Work out the finished part from the listing and answer in its coordinate system (mm). Give positions to 0.01 mm unless a question says otherwise; leave off trailing zeros. Loops run counter-clockwise (first coordinate to the right, second up) from the corner with the lowest first, then second, coordinate; pieces in that order, holes last.
from build123d import *

# Parameters (mm, degrees)
PAD013_DEPTH         = 9.4
POCKET039_DEPTH      = 100
POCKET039_DEPTH_BACK = 100
SKETCH049_R          = 2.3
POCKET040_DEPTH      = 1.101
CHAMFER010_SIZE      = 0.5


with BuildPart() as part:
    # Sketch047 (on Face1 of ShapeBinder008) → Pad013 (new body)
    with BuildSketch(Plane.XY.offset(4.85)):
        Polygon((-4.5, -10), (-5.6, -11.1), (5.6, -11.1), (4.5, -10), align=None)
    extrude(amount=-PAD013_DEPTH)

    # Sketch048 (on DatumPlane) → Pocket039 (cut, two sides)
    with BuildSketch(Plane(origin=(-4.866667, -10.366667, 1.716667), x_dir=(0, -1, 0), z_dir=(-1, 0, 0))) as pocket039_sk:
        Polygon((0.833333, 2.591912), (-0.366667, 1.391912), (-1.166667, 1.391912), (-1.166667, 3.391912), (0.833333, 3.391912), align=None)
    extrude(amount=-POCKET039_DEPTH, mode=Mode.SUBTRACT)
    extrude(pocket039_sk.sketch, amount=POCKET039_DEPTH_BACK, mode=Mode.SUBTRACT)

    # Sketch049 (on Face5 of Pocket039) → Pocket040 (cut, through all)
    with BuildSketch(Plane(origin=(0, -10, 0), x_dir=(-1, 0, 0), z_dir=(0, 1, 0))):
        with Locations((0, 1.15)):
            Circle(SKETCH049_R)
    extrude(amount=-POCKET040_DEPTH, mode=Mode.SUBTRACT)

    # Chamfer010
    chamfer010_edges = [part.edges().sort_by_distance(p)[0] for p in [
        (0, -10, -4.55),
    ]]
    chamfer(chamfer010_edges, length=CHAMFER010_SIZE)


solid = part.part
Item 1: Find section B-B, the plane x = 0.75. Write down the section's boundary in (y, z), plus the area to 3 significant figures.
Item 2: Determine the mould class of faces 1 (the face through (0.499, -10.542, -1.095)), 2 (the face through (1.1, -10, -1.2)), 3 (the face through (5.1, -10.6, -0.1)) for opening direction X: released by +X, released by -X, zero draft, split by the parting line, or undercut.
Item 3: Find section C-C, the plane y = -10.95. Write down the section's boundary in (x, z), plus the area to 3 significant figures.
Item 4: Consider line 1 (X direction, y = -10.5, z = 1.15); line 2 (Z direction, x = 0, y = -10.75); line 3 (X direction, y = -10.85, z = 1.15). Determine where each line is inside the solid, lowest interval first.
Item 5: Find section D-D, the plane x = -4. Write down the section's boundary in (y, z).
Item 6: Find section A-A, the plane z = 1.15. Write down the section's boundary in (x, y), plus the area to 3 significant figures.
Ans:
1. outline: (-11.1, -4.55) - (-10.5, -4.55) - (-10, -4.05) - (-10, -1.02) - (-11.1, -1.02) - close; (-11.1, 3.32) - (-10.22, 3.32) - (-11.1, 4.21) - close
1. area: 4.14 mm2
2. face 1: undercut
2. face 2: zero draft
2. face 3: released by +X
3. outline: (-5.45, -4.55) - (5.45, -4.55) - (5.45, 4.06) - (-5.45, 4.06) - close; hole circle Ø4.6 at (0, 1.15)
3. area: 77.2 mm2
4. line 1: x = -5 to -2.3, 2.3 to 5
4. line 2: z = -4.55 to -1.15, 3.45 to 3.86
4. line 3: x = -5.35 to -2.3, 2.3 to 5.35
5. outline: (-11.1, -4.55) - (-10.5, -4.55) - (-10, -4.05) - (-10, 3.11) - (-11.1, 4.21) - close
6. outline: (-5.6, -11.1) - (-2.3, -11.1) - (-2.3, -10) - (-4.5, -10) - close; (2.3, -11.1) - (5.6, -11.1) - (4.5, -10) - (2.3, -10) - close
6. area: 6.05 mm2
